```python
from build123d import *

# Parameters (mm, degrees)
F1_DEPTH = 250


with BuildPart() as f1:
    # F0 (on Front) → F1 (new body)
    with BuildSketch(Plane.XZ):
        Polygon((3, 3), (7.5, 3), (3, 6.5), align=None)
        Polygon((-3, 6.5), (-7.5, 3), (-3, 3), align=None)
        Polygon((-3, 10), (0, 10), (0, 15.5), (-11, 15.5), (-11, 10), align=None)
        Polygon((0, 15.5), (0, 10), (3, 10), (11, 10), (11, 15.5), align=None)
        Polygon((0, 0), (7.5, 0), (7.5, 3), (3, 3), (0, 3), align=None)
        Polygon((-7.5, 0), (0, 0), (0, 3), (-3, 3), (-7.5, 3), align=None)
        Polygon((-3, 3), (0, 3), (0, 10), (-3, 10), (-3, 6.5), align=None)
        Polygon((0, 10), (0, 3), (3, 3), (3, 6.5), (3, 10), align=None)
    extrude(amount=F1_DEPTH)


solid = f1.part
```
The listing builds one solid part. Answer for the finished solid, in the listing's coordinates (mm). A direction names the side the tool comes from. Give positions to 0.01 mm unless a question says otherwise; leave off trailing zeros. Loops run counter-clockwise (first coordinate to the right, second up) from the corner with the lowest first, then second, coordinate; pieces in that order, holes last. Notation, with made-up numbers: (-24, 2.25) - (-15, 2.25) arc R32 cw to (-15, 41.25) - close; hole circle Ø8 at (-31.75, 47). An arc over 180 degrees is marked (long way). Return JSON: item names as keys, results as strings. Group by question number.
1. Determine the mould class of faces 1 (the flat face through (0, -123, 0)), 2 (the flat face through (0, -250, 8)), 3 (the flat face through (-7, -123, 10)) for opening direction Z: pulls with the +Z half, pulls with the -Z half, needs draft (parallel to the pull), parting line crosses it, or undercut.
2. Find section A-A (y = -147). Write down the section's boundary in (x, z).
3. Given pin 1 Ø1.8 at (y, z) = (-137.5, 9) entering from +X; pin 2 Ø2.5 at (y, z) = (-64.5, 1) entering from +X; pin 3 Ø2.5 at (y, z) = (-93.5, 2) entering from -X, each flat-ended and moving along its own axis, determine where each tip first touches the part or whether it passes through.
4. Straight lines are drawn through the part: line 1 (X direction, y = -120, z = 9); line 2 (Z direction, x = -3.75, y = -210.5); line 3 (Z direction, x = 6.5, y = -96). For each, find the intervals that lie inside material, in ascending order. Write a range as [from, to].
5. Which of the six approach directions +Z, -Z, +X, -X, +Y, -Y give full straight-line access (tool end or side, diameter ignored) to faces 4 (the flat face through (5.281, -123.25, 4.726)), 5 (the flat face through (-11, -123, 13)), 6 (the flat face through (-5.219, -123.25, 4.774))?
Verdict:
{
 "1": {"face 1": "pulls with the -Z half", "face 2": "needs draft", "face 3": "undercut"},
 "2": {"outline": "(-11, 10) - (-3, 10) - (-3, 6.5) - (-7.5, 3) - (-7.5, 0) - (7.5, 0) - (7.5, 3) - (3, 6.5) - (3, 10) - (11, 10) - (11, 15.5) - (-11, 15.5) - close"},
 "3": {"pin 1": "stops at x = 3", "pin 2": "stops at x = 7.5", "pin 3": "stops at x = -7.5"},
 "4": {"line 1": "x = [-3, 3]", "line 2": "z = [0, 5.92], [10, 15.5]", "line 3": "z = [0, 3.78], [10, 15.5]"},
 "5": {"face 4": "+X, +Y, -Y", "face 5": "+Z, -Z, -X, +Y, -Y", "face 6": "-X, +Y, -Y"}
}
